The listing builds one solid part. Answer for the finished solid, in the listing's coordinates (mm). Face numbers are marked on the shaded views. Give positions to 0.01 mm unless a question says otherwise; leave off trailing zeros. Write each loop counter-clockwise with the first axis right and the second up, starting at its lowest first coordinate (ties: lowest second). Pieces come first, ordered by that corner, then holes. Notation, with made-up numbers: (2, -4) -> (36, -4) arc R10 cw to (36, 15) -> close; hole circle Ø5 at (6.5, -10.75). An arc over 180 degrees is marked (long way). Use CSV: the item, a comma, the result in double quotes. Start each with the question number.
from build123d import *

# Parameters (mm, degrees)
SKETCH2_W                    = 75
SKETCH2_H                    = 100
BOSS_EXTRUDE1_DEPTH          = 10
BOSS_EXTRUDE4_DEPTH          = 10
F_5_0_5_DIAMETER_HOLE1_D     = 5
CUT_EXTRUDE1_DEPTH           = 6
FILLET1_R                    = 10
F_3_0_3_DIAMETER_HOLE1_D     = 3
F_3_0_3_DIAMETER_HOLE1_DEPTH = 10
F_3_0_3_DIAMETER_HOLE1_TIP   = 0.901290929
SKETCH18_W                   = 17
SKETCH18_H                   = 8
BOSS_EXTRUDE5_DEPTH          = 3
FILLET2_R                    = 4
CUT_EXTRUDE2_DEPTH           = 10
CHAMFER1_SIZE                = 2


with BuildPart() as part:
    # Sketch2 → Boss-Extrude1 (new body)
    with BuildSketch(Plane.XY):
        with Locations((37.5, 50)):
            Rectangle(SKETCH2_W, SKETCH2_H)
    extrude(amount=BOSS_EXTRUDE1_DEPTH)

    # Sketch5 → Boss-Extrude4 (add)
    with BuildSketch(Plane.XY.offset(10)):
        with BuildLine():
            ThreePointArc((25.222170949, 60.16471593), (40, 15), (54.777829051, 60.16471593))
            ThreePointArc((54.777829051, 60.16471593), (51.923594578, 61.973345042), (48.851534275, 63.380554762))
            ThreePointArc((48.851534275, 63.380554762), (40, 65), (31.148465725, 63.380554762))
            ThreePointArc((31.148465725, 63.380554762), (28.076405422, 61.973345042), (25.222170949, 60.16471593))
        make_face()
    extrude(amount=BOSS_EXTRUDE4_DEPTH)

    # Ø5.0 (5) Diameter Hole1 (through all)
    with Locations(Plane.XY.offset(20)):
        with Locations((31.161165235, 48.838834765), (48.838834765, 48.838834765)):
            Hole(F_5_0_5_DIAMETER_HOLE1_D / 2)

    # Sketch12 → Cut-Extrude1 (cut)
    with BuildSketch(Plane.XY.offset(10)):
        with BuildLine():
            Line((15, 89), (65, 89))
            ThreePointArc((65, 89), (69, 85), (65, 81))
            Line((65, 81), (15, 81))
            ThreePointArc((15, 81), (11, 85), (15, 89))
        make_face()
    extrude(amount=-CUT_EXTRUDE1_DEPTH, mode=Mode.SUBTRACT)

    # Fillet1
    fillet1_edges = [part.edges().sort_by_distance(p)[0] for p in [
        (0, 100, 5),
        (75, 100, 5),
        (75, 0, 5),
        (0, 0, 5),
    ]]
    fillet(fillet1_edges, radius=FILLET1_R)

    # Ø3.0 (3) Diameter Hole1
    with Locations(Plane.XY.offset(10)):
        with Locations((15, 73), (37.5, 73)):
            Hole(F_3_0_3_DIAMETER_HOLE1_D / 2, depth=F_3_0_3_DIAMETER_HOLE1_DEPTH)
            with Locations((0, 0, -(F_3_0_3_DIAMETER_HOLE1_DEPTH + F_3_0_3_DIAMETER_HOLE1_TIP / 2))):  # 118° drill point
                Cone(0, F_3_0_3_DIAMETER_HOLE1_D / 2, F_3_0_3_DIAMETER_HOLE1_TIP, mode=Mode.SUBTRACT)

    # Sketch18 → Boss-Extrude5 (add)
    with BuildSketch(Plane.XY.offset(4)):
        with Locations((43.5, 85)):
            Rectangle(SKETCH18_W, SKETCH18_H)
    extrude(amount=BOSS_EXTRUDE5_DEPTH)

    # Fillet2
    fillet2_edges = [part.edges().sort_by_distance(p)[0] for p in [
        (52, 81, 5.5),
        (52, 89, 5.5),
        (35, 81, 5.5),
        (35, 89, 5.5),
    ]]
    fillet(fillet2_edges, radius=FILLET2_R - 0.0001)  # a hair under: the kernel refuses the full size

    # Sketch20 → Cut-Extrude2 (cut)
    with BuildSketch(Plane.XY.offset(20)):
        with BuildLine():
            ThreePointArc((54.498623519, 31.756776834), (40, 40.773853631), (25.501376481, 31.756776834))
            ThreePointArc((25.501376481, 31.756776834), (27.320380503, 26.400357846), (32.67679949, 28.219361868))
            ThreePointArc((32.67679949, 28.219361868), (40, 32.773853631), (47.32320051, 28.219361868))
            ThreePointArc((47.32320051, 28.219361868), (52.679619497, 26.400357846), (54.498623519, 31.756776834))
        make_face()
    extrude(amount=-CUT_EXTRUDE2_DEPTH, mode=Mode.SUBTRACT)

    # Chamfer1
    chamfer1_edges = [part.edges().sort_by_distance(p)[0] for p in [
        (25.222170949, 19.83528407, 20),
    ]]
    chamfer(chamfer1_edges, length=CHAMFER1_SIZE)


solid = part.part
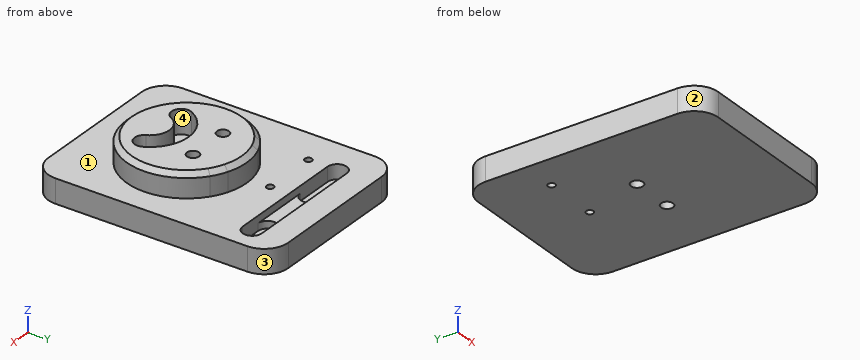
Q1. The mould has two halves that part along Y. Classify the marked faces 1, 2, 3 and 4: +Y half, -Y half, draft (parallel to the pull), parting line (faces both ways), or undercut.
Q2. Section B-B on z = 12.5 is taken. Give the vertices of the cut face in (x, y).
Q3. Flat-ended cylindrical pins translate along their axes: pin 1 Ø2 at (x, y) = (37, 83) entering from +Z; pin 2 Ø10 at (x, y) = (42.5, 83.5) entering from +Z; pin 3 Ø4 at (x, y) = (23.5, 84) entering from +Z; pin 4 Ø4 at (x, y) = (48.84, 48.84) entering from -Z. Find the tip coordinate at first contact, or state that the pin passes through.
Q4. Straight lines are drawn through the part: L1, parallel to Y at x = 31, z = 4.5; L2, parallel to X at y = 73, z = 6.25; L3, parallel to Y at x = 15, z = 7.75. For each, find the intervals that lie inside material, in ascending order.
Q5. Section A-A on y = 73 is taken. Give the vertices of the cut face in (x, z), then the cut area to 3 significant figures.
Output:
1,face 1,"draft"
1,face 2,"-Y half"
1,face 3,"+Y half"
1,face 4,"undercut"
2,outline,"circle Ø50 at (40, 40); hole (25.5, 31.76) arc R4 ccw to (32.68, 28.22) arc R8.16 cw to (47.32, 28.22) arc R4 ccw to (54.5, 31.76) arc R16.16 ccw to start; hole circle Ø5 at (31.16, 48.84); hole circle Ø5 at (48.84, 48.84)"
3,pin 1,"z = 7"
3,pin 2,"z = 10"
3,pin 3,"z = 4"
3,pin 4,"through"
4,L1,"0 to 46.34, 51.33 to 81, 89 to 100"
4,L2,"0 to 13.5, 16.5 to 36, 39 to 75"
4,L3,"0 to 71.5, 74.5 to 81, 89 to 100"
5,outline,"(0, 0) -> (13.5, 0) -> (13.5, 10) -> (0, 10) -> close; (16.5, 0) -> (36, 0) -> (36, 10) -> (16.5, 10) -> close; (39, 0) -> (75, 0) -> (75, 10) -> (39, 10) -> close"
5,area,"690 mm²"
